Drawing for the job (mm, zero at the part's lowest x, y, z). Coordinates: 2 decimals unless noted, no trailing zeros. Write each loop counter-clockwise with the first axis right and the second up, starting at its lowest first coordinate (ties: lowest second). Pieces come first, ordered by that corner, then holes. Notation, with made-up numbers: M 24,78 L 80,78 A20 ccw 80,95 Z; hole C -1,-10.75 d2. An arc over 180 degrees is marked long. Put each result on its own line as item: value. Start each with the question number.
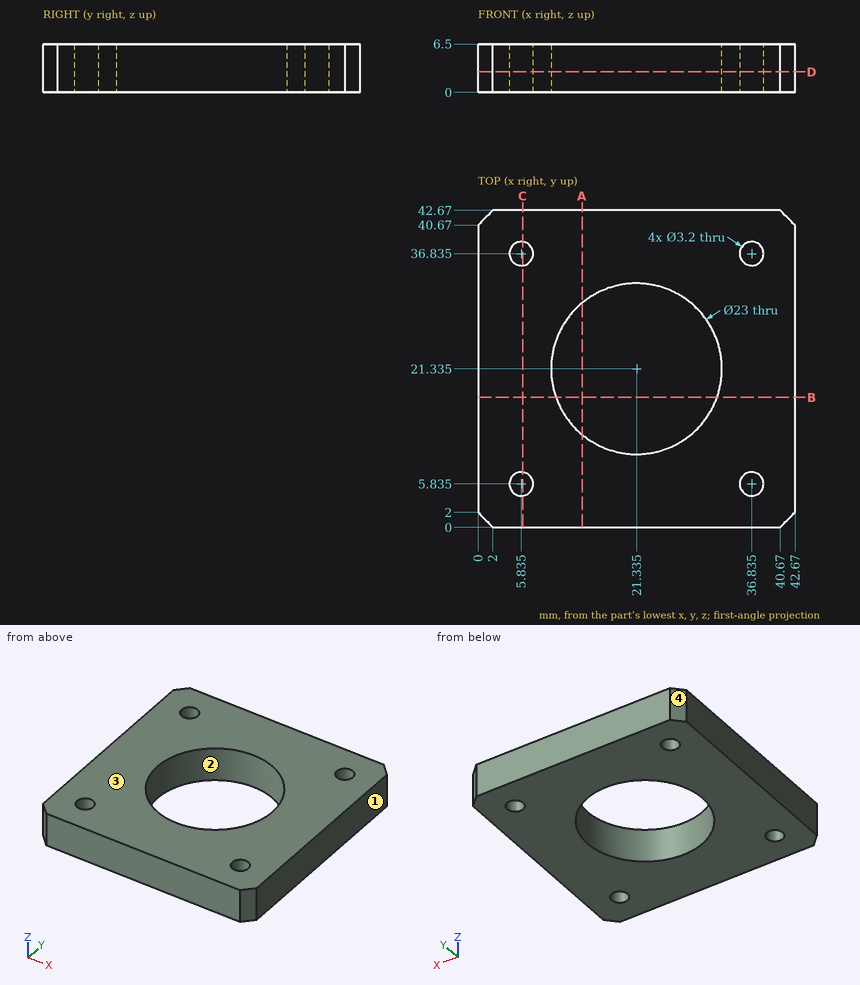
(1) Two-plate mould, pull along X, no slides. Class the marked faces 1, 2, 3 and 4: +X half, -X half, draft (parallel to the pull), parting line (faces both ways), or undercut.
(2) Slice it at C-C, the plane x = 6. Write the cut outline in (y, z).
(3) Slice it at B-B, the plane y = 17.5. Write the cut outline in (x, z), then the cut area to 3 significant figures.
(4) Slice it at A-A, the plane x = 14. Write the cut outline in (y, z).
(5) Drill centre lines: line 1 (Y direction, x = 35.5, z = 2); line 2 (X direction, y = 22, z = 4); line 3 (Y direction, x = 16, z = 3). Where is each one in solid material? Low to high. Write a range as [from, to].
(6) Slice it at D-D, the plane z = 2.75. Write the cut outline in (x, y) (3 decimals), then the cut area to 3 significant figures.
Result set:
1. face 1: +X half
1. face 2: undercut
1. face 3: draft
1. face 4: -X half
2. outline: M 0,0 L 4.24,0 L 4.24,6.5 L 0,6.5 Z; M 7.43,0 L 35.24,0 L 35.24,6.5 L 7.43,6.5 Z; M 38.43,0 L 42.67,0 L 42.67,6.5 L 38.43,6.5 Z
3. outline: M 0,0 L 10.49,0 L 10.49,6.5 L 0,6.5 Z; M 32.18,0 L 42.67,0 L 42.67,6.5 L 32.18,6.5 Z
3. area: 136 mm^2
4. outline: M 0,0 L 12.48,0 L 12.48,6.5 L 0,6.5 Z; M 30.19,0 L 42.67,0 L 42.67,6.5 L 30.19,6.5 Z
5. line 1: y = [0, 4.95], [6.72, 35.95], [37.72, 42.67]
5. line 2: x = [0, 9.85], [32.82, 42.67]
5. line 3: y = [0, 11.15], [31.52, 42.67]
6. outline: M 0,2 L 2,0 L 40.67,0 L 42.67,2 L 42.67,40.67 L 40.67,42.67 L 2,42.67 L 0,40.67 Z; hole C 5.835,5.835 d3.2; hole C 5.835,36.835 d3.2; hole C 21.335,21.335 d23; hole C 36.835,5.835 d3.2; hole C 36.835,36.835 d3.2
6. area: 1,370 mm^2
